Work out the finished part from the listing and answer in its coordinate system (mm). A direction names the side the tool comes from. Round coordinates to 2 decimals unless told otherwise and drop trailing zeros. Order: outer loops, then holes, each group sorted by start corner. A loop starts at its lowest first (then second) coordinate and runs counter-clockwise, first axis right, second up. Notation, with made-up numbers: (14, 78) - (23, 78) arc R28 cw to (23, 101) - close; hole circle Ø2 at (82, 6). An arc over 180 degrees is marked (long way). Put each result on its own line as item: value.
```python
from build123d import *

# Parameters (mm, degrees)
ESBO_O2_R                = 25
ESBO_O3_R                = 6
RESSALTO_EXTRUS_O1_DEPTH = 35
ESBO_O4_R                = 6
CORTE_EXTRUS_O1_DEPTH    = 20


with BuildPart() as part:
    # Varredura1: sweep along a path in Esboço1
    with BuildLine(Plane.XY) as varredura1_path:
        Line((16.90473047, 76.252311481), (0, 40))
        Line((0, 40), (0, 0))
    # Esboço2 → Varredura1 (sweep)
    with BuildSketch(Plane(origin=(0, 0, 0), x_dir=(1, 0, 0), z_dir=(0, 1, 0))):
        Circle(ESBO_O2_R)
    sweep(path=varredura1_path.line, transition=Transition.RIGHT)

    # Esboço3 → Ressalto-extrusão1 (add)
    with BuildSketch(Plane(origin=(32.225619332, 69.108063675, 0), x_dir=(0.906307787, -0.422618262, 0), z_dir=(0.422618262, 0.906307787, 0))):
        with Locations((-16.90473047, 0)):
            Circle(ESBO_O3_R)
    extrude(amount=RESSALTO_EXTRUS_O1_DEPTH)

    # Esboço4 → Corte-extrusão1 (cut)
    with BuildSketch(Plane.XZ):
        Circle(ESBO_O4_R)
    extrude(amount=-CORTE_EXTRUS_O1_DEPTH, mode=Mode.SUBTRACT)


solid = part.part
```
1) A cutting plane is placed at C-C on y = 33. Write down the section's boundary in (x, z).
Findings below:
outline: circle Ø50 at (0, 0)
2) Given pin 1 Ø1.5 at (y, z) = (51.5, -13) entering from -X; pin 2 Ø19 at (x, z) = (0, 0) entering from -Y; pin 3 Ø5 at (y, z) = (32.5, -9.5) entering from +X; pin 4 Ø1 at (x, y) = (-18, 47) entering from -Z, each flat-ended and moving along its own axis, determine where each tip first touches the part or whether it passes through.
Findings below:
pin 1: stops at x = -18.8
pin 2: stops at y = 0
pin 3: stops at x = 24
pin 4: stops at z = -16.51
3) A cutting plane is placed at B-B on y = 9.5. Write down the section's boundary in (x, z).
Findings below:
outline: circle Ø50 at (0, 0); hole circle Ø12 at (0, 0)
4) A cutting plane is placed at D-D on z = -16. Write down the section's boundary in (x, y), then the cut area to 3 significant figures.
Findings below:
outline: (-19.21, 0) - (19.21, 0) - (19.21, 35.74) - (34.31, 68.13) - (-0.5, 84.37) - (-19.21, 44.26) - close
area: 3,070 mm2
5) Straight lines are drawn through the part: L1, parallel to Z at x = 0, y = 6.25; L2, parallel to Z at x = -3, y = 10.5; L3, parallel to Y at x = 11, z = 8. For each, find the intervals that lie inside material, in ascending order. Write a range as from..to.
Findings below:
L1: z = -25..-6, 6..25
L2: z = -24.82..-5.2, 5.2..24.82
L3: y = 0..79.01
6) For faces 4 (the flat face through (31.62, 108.01, -0.08)), 5 (the flat face through (0, 20, 0)), 6 (the flat face through (21.623, 74.052, 5.206)), determine the directions among +Z, -Z, +X, -X, +Y, -Y from which every point of the face is accessible in a straight line to the end or side of a thin tool.
Findings below:
face 4: +Z, -Z, +X, +Y
face 5: -Y
face 6: none
7) For a pull along X with two mould halves and no side action, classify faces 1 (the cylindrical face through (-13.35, 70.47, 1.1)), 2 (the cylindrical face through (-6, 10, 0)), 3 (the flat face through (-5, 0, 5)) as pulls with the +X half, pulls with the -X half, needs draft (parallel to the pull), parting line crosses it, or undercut.
Findings below:
face 1: parting line crosses it
face 2: undercut
face 3: needs draft
8) A cutting plane is placed at A-A on z = 3. Write down the section's boundary in (x, y), then the cut area to 3 significant figures.
Findings below:
outline: (-24.82, 0) - (-5.2, 0) - (-5.2, 20) - (5.2, 20) - (5.2, 0) - (24.82, 0) - (24.82, 34.5) - (39.4, 65.76) - (21.61, 74.06) - (36.41, 105.78) - (26.99, 110.17) - (12.2, 78.45) - (-5.59, 86.74) - (-24.82, 45.5) - close
area: 4,130 mm2
